Read the model definition and answer for the solid it produces. Units are mm, in the model's axes. Face numbers are marked on the shaded views. A direction names the side the tool comes from. Round coordinates to 2 decimals unless told otherwise and drop trailing zeros. Loops run counter-clockwise (first coordinate to the right, second up) from the corner with the lowest first, then second, coordinate; pieces in that order, holes last. Notation, with made-up numbers: M 70,67.25 L 77,67.25 A21 cw 77,91.25 Z; hole C -9.75,82.25 d3. An arc over 180 degrees is marked long. Write each question's results on one line, items separated by ' | '.
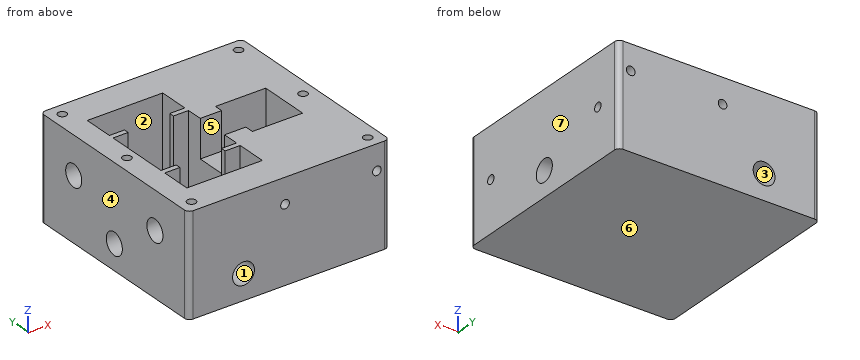
from build123d import *

# Parameters (mm, degrees)
F1_DEPTH  = 40
F2_W      = 20
F2_H      = 20
F3_DEPTH  = 35
F4_R      = 4.35
F5_DEPTH  = 15
F6_R      = 4.35
F7_DEPTH  = 15
F8_W      = 8.4756634911
F8_H      = 13.160008005
F9_DEPTH  = 15
F10_R     = 1.725
F11_DEPTH = 15
F12_R     = 11.5
F13_DEPTH = 2.5
F14_R     = 1.725
F15_DEPTH = 10
F16_R     = 1.725
F17_DEPTH = 10
F18_R     = 1.725
F19_DEPTH = 25
F20_R     = 4.35
F21_DEPTH = 15
F22_R     = 4.35
F23_DEPTH = 15
F24_W     = 18
F24_H     = 2
F25_DEPTH = 6


# Not quite as in the source:
# - a feature names something its author has since deleted; it is built from what else it names


with BuildPart() as f1:
    # F0 (on Top) → F1 (new body)
    with BuildSketch(Plane.XY):
        with BuildLine():
            ThreePointArc((40, 38), (39.4142135624, 39.4142135624), (38, 40))
            Line((38, 40), (-38, 40))
            ThreePointArc((-38, 40), (-39.4142135624, 39.4142135624), (-40, 38))
            Line((-40, 38), (-40, -38))
            ThreePointArc((-40, -38), (-39.4142135624, -39.4142135624), (-38, -40))
            Line((-38, -40), (38, -40))
            ThreePointArc((38, -40), (39.4142135624, -39.4142135624), (40, -38))
            Line((40, -38), (40, 38))
        make_face()
    extrude(amount=F1_DEPTH)

    # F2 (on face) → F3 (cut)
    with BuildSketch(Plane.XY.offset(40)):
        with Locations((17.50956662, 0)):
            Rectangle(F2_W, F2_H)
        Polygon((-24.9660968933, -15), (-30.9660968933, -15), (-30.9660968933, -26.9999999998), (-0.9660968933, -26.9999999998), (-0.9660968933, -15), (-6.9660968933, -15), (-6.9660968933, -13), (-0.9660968933, -13), (-0.9660968933, 13), (-6.9660968933, 13), (-6.9660968933, 15), (-0.9660968933, 15), (-0.9660968933, 26.9999999998), (-30.9660968933, 26.9999999998), (-30.9660968933, 15), (-24.9660968933, 15), (-24.9660968933, 13), (-30.9660968933, 13), (-30.9660968933, -13), (-24.9660968933, -13), align=None)
    extrude(amount=-F3_DEPTH, mode=Mode.SUBTRACT)

    # F4 (on face) → F5 (cut)
    with BuildSketch(Plane(origin=(-40, 0, 0), x_dir=(0, -1, 0), z_dir=(-1, 0, 0))):
        with Locations((-22, 25)):
            Circle(F4_R)
        with Locations((22, 25)):
            Circle(F4_R)
        with Locations((0, 10)):
            Circle(F4_R)
    extrude(amount=-F5_DEPTH, mode=Mode.SUBTRACT)

    # F6 (on face) → F7 (cut)
    with BuildSketch(Plane.YZ.offset(40)):
        with Locations((0, 10)):
            Circle(F6_R)
    extrude(amount=-F7_DEPTH, mode=Mode.SUBTRACT)

    # F8 (on face) → F9 (cut)
    with BuildSketch(Plane.XY.offset(40)):
        with Locations((3.2717348745, 0.0860663135)):
            Rectangle(F8_W, F8_H)
    extrude(amount=-F9_DEPTH, mode=Mode.SUBTRACT)

    # F10 (on face) → F11 (cut)
    with BuildSketch(Plane.XY.offset(40)):
        with Locations((-35, 0)):
            Circle(F10_R)
        with Locations((35, 0)):
            Circle(F10_R)
        with Locations((-35, 35)):
            Circle(F10_R)
        with Locations((-35, -35)):
            Circle(F10_R)
        with Locations((35, 35)):
            Circle(F10_R)
        with Locations((35, -35)):
            Circle(F10_R)
    extrude(amount=-F11_DEPTH, mode=Mode.SUBTRACT)

    # F12 (on face) → F13 (cut)
    with BuildSketch(Plane.XY.offset(5)):
        with Locations((-15.966096893, 0)):
            Circle(F12_R)
    extrude(amount=-F13_DEPTH, mode=Mode.SUBTRACT)

    # F14 (on face) → F15 (cut)
    with BuildSketch(Plane.XZ.offset(40)):
        with Locations((-1.5, 30)):
            Circle(F14_R)
        with Locations((35, 30)):
            Circle(F14_R)
    extrude(amount=-F15_DEPTH, mode=Mode.SUBTRACT)

    # F16 (on face) → F17 (cut)
    with BuildSketch(Plane(origin=(0, 40, 0), x_dir=(-1, 0, 0), z_dir=(0, 1, 0))):
        with Locations((-35, 30)):
            Circle(F16_R)
        with Locations((1.5, 30)):
            Circle(F16_R)
    extrude(amount=-F17_DEPTH, mode=Mode.SUBTRACT)

    # F18 (on face) → F19 (cut)
    with BuildSketch(Plane.YZ.offset(40)):
        with Locations((-29, 20)):
            Circle(F18_R)
        with Locations((29, 20)):
            Circle(F18_R)
    extrude(amount=-F19_DEPTH, mode=Mode.SUBTRACT)

    # F20 (on face) → F21 (cut)
    with BuildSketch(Plane(origin=(0, 40, 0), x_dir=(-1, 0, 0), z_dir=(0, 1, 0))):
        with Locations((18, 10)):
            Circle(F20_R)
    extrude(amount=-F21_DEPTH, mode=Mode.SUBTRACT)

    # F22 (on face) → F23 (cut)
    with BuildSketch(Plane.XZ.offset(40)):
        with Locations((-18, 10)):
            Circle(F22_R)
    extrude(amount=-F23_DEPTH, mode=Mode.SUBTRACT)

    # F24 (on face) → F25 (join)
    with BuildSketch(Plane.XY.offset(5)):
        with Locations((-15.9660968933, 14)):
            Rectangle(F24_W, F24_H)
        with Locations((-15.9660968933, -14)):
            Rectangle(F24_W, F24_H)
    extrude(amount=F25_DEPTH)


solid = f1.part
Item 1: Straight lines are drawn through the part: line 1 (Y direction, x = -5.5, z = 33.5); line 2 (X direction, y = 7.5, z = 15.5); line 3 (Y direction, x = -35, z = 34) (3 decimals). For each, find the intervals that lie inside material, in ascending order.
Outcome:
line 1: y = -40 to -27, -15 to -13, 13 to 15, 27 to 40 | line 2: x = -40 to -30.97, -0.97 to 7.51, 27.51 to 40 | line 3: y = -40 to -36.725, -33.275 to -1.725, 1.725 to 33.275, 36.725 to 40
Item 2: The part is cut by section D-D (y = 0). State how many separate pieces and enclosed holes the cut face has, plus the area to 3 significant figures.
Outcome:
separate pieces: 3 | enclosed holes: 0 | area: 975 mm2
Item 3: For the marked faces 1, 2, 3 and 4, determine the directions among +Z, -Z, +X, -X, +Y, -Y from which every point of the face is accessible in a straight line to the end or side of a thin tool.
Outcome:
face 1: -Y | face 2: +Z | face 3: +Y | face 4: +Z, -Z, -X, +Y, -Y
Item 4: Flat-ended cylindrical pins translate along their axes: pin 1 (2 mm diameter, centred on x = -1.5, z = 30, fed in from -Y); pin 2 (1 mm diameter, centred on x = -35.5, y = -35.5, fed in from +Z); pin 3 (5 mm diameter, centred on x = -10, y = -20, fed in from +Z); pin 4 (16 mm diameter, centred on x = 16, y = -5, fed in from +Z). Find the tip coordinate at first contact, or state that the pin passes through.
Outcome:
pin 1: stops at y = -30 | pin 2: stops at z = 25 | pin 3: stops at z = 5 | pin 4: stops at z = 40
Item 5: The part is cut by section B-B (y = -22). Determine the outline of the cut face in (x, z), plus the area to 3 significant figures.
Outcome:
outline: M -40,0 L 40,0 L 40,40 L -0.97,40 L -0.97,5 L -30.97,5 L -30.97,20.65 L -40,20.65 Z; M -40,29.35 L -30.97,29.35 L -30.97,40 L -40,40 Z | area: 2,070 mm2
Item 6: The mould has two halves that part along X. Classify the marked faces 5, 6 and 7: pulls with the +X half, pulls with the -X half, needs draft (parallel to the pull), parting line crosses it, or undercut.
Outcome:
face 5: undercut | face 6: needs draft | face 7: pulls with the +X half
Item 7: The part is cut by section A-A (x = -35). Determine the outline of the cut face in (y, z) (3 decimals).
Outcome:
outline: M -40,0 L 40,0 L 40,40 L 36.725,40 L 36.725,25 L 33.275,25 L 33.275,40 L 1.725,40 L 1.725,25 L -1.725,25 L -1.725,40 L -33.275,40 L -33.275,25 L -36.725,25 L -36.725,40 L -40,40 Z; hole C -22,25 d8.7; hole C 0,10 d8.7; hole C 22,25 d8.7
Item 8: The part is cut by section C-C (x = 18). Determine the outline of the cut face in (y, z) (3 decimals), plus the area to 3 significant figures.
Outcome:
outline: M -40,0 L 40,0 L 40,40 L 10,40 L 10,5 L -10,5 L -10,40 L -40,40 Z; hole C -29,20 d3.45; hole C 29,20 d3.45 | area: 2,480 mm2
